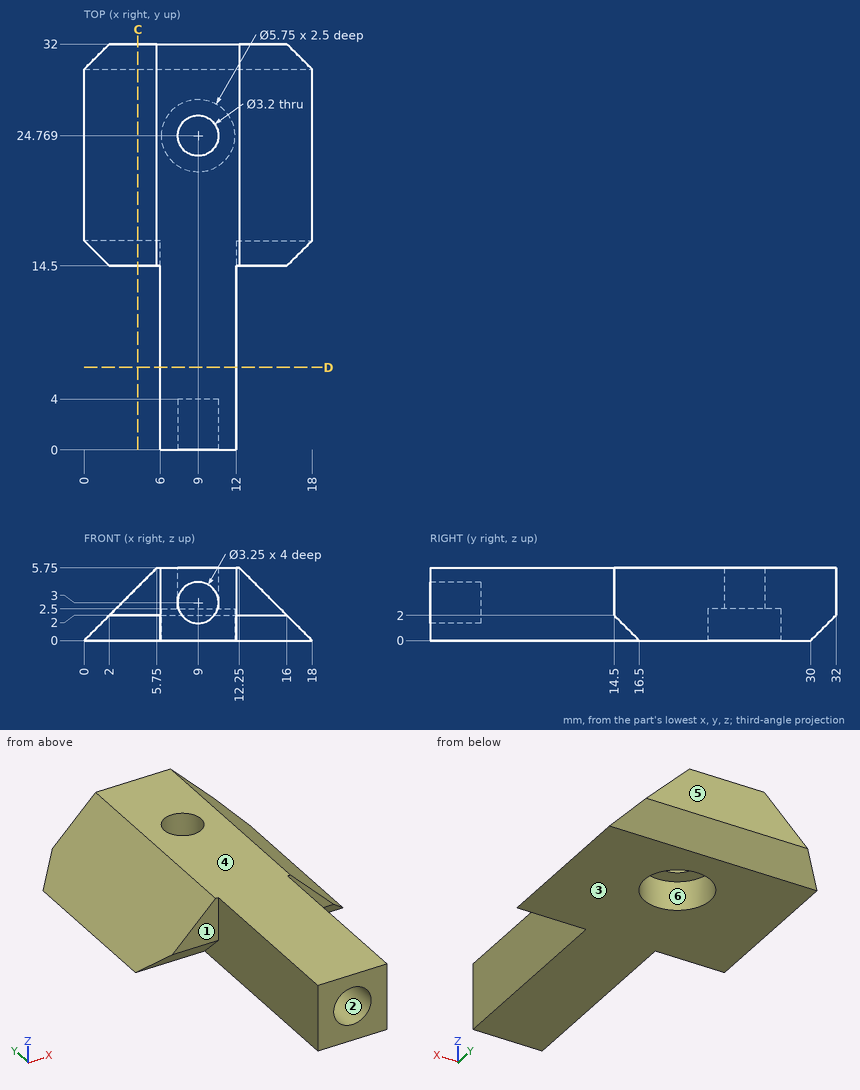
Part print with two shaded views. Sizes in mm from the minimum x, y, z corner. A direction names the side the tool comes from. Give positions to 0.01 mm unless a question says otherwise; leave off trailing zeros. Order: outer loops, then holes, each group sorted by start corner. A loop starts at its lowest first (then second) coordinate and runs counter-clockwise, first axis right, second up.
(1) Saw through at C-C, the plane x = 4.25. Give the cut face in (y, z).
(2) Drill centre lines: L1, parallel to Y at x = 9, z = 3.3; L2, parallel to Y at x = 12.25, z = 2.2; L3, parallel to Z at x = 7.5, y = 23.5. Where is each one in solid material? Low to high.
(3) Flat gauge pins, fed straight in: pin 1 (3 mm diameter, centred on x = 9, y = 24.77, fed in from -Z); pin 2 (10 mm diameter, centred on x = 5.5, y = 26, fed in from +Z); pin 3 (1.7 mm diameter, centred on y = 9.5, z = 2.5, fed in from -X); pin 4 (1.7 mm diameter, centred on x = 9, y = 23.5, fed in from -Z). Where does each tip first touch, or does it go through?
(4) Saw through at D-D, the plane y = 6.5. Give the cut face in (x, z), then the cut area to 3 significant figures.
(5) Tool access for the marked faces 1, 2 and 3: list every direction of +Z, -Z, +X, -X, +Y, -Y with a clear straight run to the whole face (end or side of a thin tool).
(6) Mould opens along Y. For the marked faces 4, 5 and 6 say: released by +Y, released by -Y, zero draft, split by the parting line, or undercut.
Results found:
1. outline: (14.5, 2) - (16.5, 0) - (30, 0) - (32, 2) - (32, 4.25) - (14.5, 4.25) - close
2. L1: y = 4 to 23.17, 26.37 to 32
2. L2: y = 14.5 to 32
2. L3: z = 2.5 to 5.75
3. pin 1: passes through
3. pin 2: stops at z = 5.75
3. pin 3: stops at x = 6
3. pin 4: stops at z = 2.5
4. outline: (6, 0) - (12, 0) - (12, 5.75) - (6, 5.75) - close
4. area: 34.5 mm2
5. face 1: +Z, -Z, -X, -Y
5. face 2: -Y
5. face 3: -Z, +X, -X, +Y, -Y
6. face 4: zero draft
6. face 5: released by +Y
6. face 6: undercut
